Check sheet for the modelled part. Datum: model origin and axes. Units: mm. A direction names the side the tool comes from. Coordinates: 2 decimals unless noted, no trailing zeros. Order: outer loops, then holes, each group sorted by start corner. A loop starts at its lowest first (then second) coordinate and runs counter-clockwise, first axis right, second up.
from build123d import *

# Parameters (mm, degrees)
SKETCH5_W           = 107.15
SKETCH5_H           = 18.5
BOSS_EXTRUDE1_DEPTH = 107.94999
SKETCH4_W           = 77.94999
SKETCH4_H           = 77.15084
CUT_EXTRUDE1_DEPTH  = 7.5
FILLET1_R           = 5
FILLET3_R           = 20
CHAMFER1_SIZE       = 10
CHAMFER1_SIZE2      = 5
CUT_EXTRUDE2_DEPTH  = 2
FILLET4_R           = 20
FILLET5_R           = 2
CUT_EXTRUDE3_START  = -7.5
CUT_EXTRUDE3_DEPTH  = 7.5


with BuildPart() as part:
    # Sketch5 → Boss-Extrude1 (new body)
    with BuildSketch(Plane.ZY.offset(-91.769)):
        with Locations((-38.2134, -9.25)):
            Rectangle(SKETCH5_W, SKETCH5_H)
    extrude(amount=BOSS_EXTRUDE1_DEPTH)

    # Sketch4 → Cut-Extrude1 (cut)
    with BuildSketch(Plane(origin=(0, 0, 0), x_dir=(1, 0, 0), z_dir=(0, 1, 0))):
        with Locations((37.794005, 38.21298)):
            Rectangle(SKETCH4_W, SKETCH4_H)
    extrude(amount=-CUT_EXTRUDE1_DEPTH, mode=Mode.SUBTRACT)

    # Fillet1
    fillet1_edges = [part.edges().sort_by_distance(p)[0] for p in [
        (76.769, -3.75, -76.7884),
        (76.769, -3.75, 0.36244),
        (-1.18099, -3.75, 0.36244),
        (-1.18099, -3.75, -76.7884),
    ]]
    fillet(fillet1_edges, radius=FILLET1_R)

    # Fillet3
    fillet3_edges = [part.edges().sort_by_distance(p)[0] for p in [
        (-16.18099, -9.25, -91.7884),
        (-16.18099, -9.25, 15.3616),
        (91.769, -9.25, -91.7884),
        (91.769, -9.25, 15.3616),
    ]]
    fillet(fillet3_edges, radius=FILLET3_R)

    # Chamfer1
    chamfer1_edges = [part.edges().sort_by_distance(p)[0] for p in [
        (37.794005, 0, -91.7884),
        (91.769, 0, -38.2134),
        (-16.18099, 0, -38.2134),
        (37.794005, 0, 15.3616),
        (-10.323125624, 0, -85.930535624),
        (-10.323125624, 0, 9.503735624),
        (85.911135624, 0, 9.503735624),
        (85.911135624, 0, -85.930535624),
    ]]
    chamfer1_side = [part.faces().sort_by_distance(p)[0] for p in [
        (37.794005, 0, 13.840602865),
    ]]
    chamfer(chamfer1_edges, length=CHAMFER1_SIZE, length2=CHAMFER1_SIZE2, reference=chamfer1_side[0])

    # Sketch6 → Cut-Extrude2 (cut)
    with BuildSketch(Plane.XZ.offset(18.5)):
        with BuildLine():
            Line((3.81901, -91.7884), (71.769, -91.7884))
            ThreePointArc((71.769, -91.7884), (85.911135624, -85.930535624), (91.769, -71.7884))
            Line((91.769, -71.7884), (91.769, -4.6384))
            ThreePointArc((91.769, -4.6384), (85.911135624, 9.503735624), (71.769, 15.3616))
            Line((71.769, 15.3616), (3.81901, 15.3616))
            ThreePointArc((3.81901, 15.3616), (-10.323125624, 9.503735624), (-16.18099, -4.6384))
            Line((-16.18099, -4.6384), (-16.18099, -71.7884))
            ThreePointArc((-16.18099, -71.7884), (-10.323125624, -85.930535624), (3.81901, -91.7884))
        make_face()
        with BuildLine():
            Line((3.81901, -79.7884), (71.769, -79.7884))
            ThreePointArc((71.769, -79.7884), (77.425854249, -77.445254249), (79.769, -71.7884))
            Line((79.769, -71.7884), (79.769, -4.6384))
            ThreePointArc((79.769, -4.6384), (77.425854249, 1.018454249), (71.769, 3.3616))
            Line((71.769, 3.3616), (3.81901, 3.3616))
            ThreePointArc((3.81901, 3.3616), (-1.837844249, 1.018454249), (-4.18099, -4.6384))
            Line((-4.18099, -4.6384), (-4.18099, -71.7884))
            ThreePointArc((-4.18099, -71.7884), (-1.837844249, -77.445254249), (3.81901, -79.7884))
        make_face(mode=Mode.SUBTRACT)
    extrude(amount=-CUT_EXTRUDE2_DEPTH, mode=Mode.SUBTRACT)

    # Fillet4
    # the kernel refuses this fillet: 20 mm, written as the material it adds along each edge
    with BuildSketch(Plane(origin=(71.769, -16.5, -4.6384), x_dir=(1, 0, 0), z_dir=(0, 0, -1))) as fillet4_piece_1:
        with BuildLine():
            CenterArc((16.717797887, 20), FILLET4_R, 244.158067237, 25.841932763)
            Line((8, 2), (8, 0))
            Line((8, 0), (16.717797887, 0))
        make_face()
    revolve(axis=Axis((71.769, -16.5, -4.6384), (0, -1, 0)), revolution_arc=90)
    with BuildSketch(Plane(origin=(79.769, -16.5, -71.7884), x_dir=(1, 0, 0), z_dir=(0, 0, 1)), Plane(origin=(-4.18099, -16.5, -4.6384), x_dir=(-1, 0, 0), z_dir=(0, 0, -1))) as fillet4_piece_2:
        with BuildLine():
            CenterArc((8.717797887, -20), FILLET4_R, 90, 25.841932763)
            Line((0, -2), (0, 0))
            Line((0, 0), (8.717797887, 0))
        make_face()
    extrude(amount=67.15)
    with BuildSketch(Plane(origin=(71.769, -16.5, -71.7884), x_dir=(0, 0, -1), z_dir=(-1, 0, 0))) as fillet4_piece_3:
        with BuildLine():
            CenterArc((16.717797887, 20), FILLET4_R, 244.158067237, 25.841932763)
            Line((8, 2), (8, 0))
            Line((8, 0), (16.717797887, 0))
        make_face()
    revolve(axis=Axis((71.769, -16.5, -71.7884), (0, -1, 0)), revolution_arc=90)
    with BuildSketch(Plane(origin=(3.81901, -16.5, -79.7884), x_dir=(0, 0, -1), z_dir=(1, 0, 0)), Plane(origin=(71.769, -16.5, 3.3616), x_dir=(0, 0, 1), z_dir=(-1, 0, 0))) as fillet4_piece_4:
        with BuildLine():
            CenterArc((8.717797887, -20), FILLET4_R, 90, 25.841932763)
            Line((0, -2), (0, 0))
            Line((0, 0), (8.717797887, 0))
        make_face()
    extrude(amount=67.94999)
    with BuildSketch(Plane(origin=(3.81901, -16.5, -71.7884), x_dir=(-1, 0, 0), z_dir=(0, 0, 1))) as fillet4_piece_5:
        with BuildLine():
            CenterArc((16.717797887, 20), FILLET4_R, 244.158067237, 25.841932763)
            Line((8, 2), (8, 0))
            Line((8, 0), (16.717797887, 0))
        make_face()
    revolve(axis=Axis((3.81901, -16.5, -71.7884), (0, -1, 0)), revolution_arc=90)
    with BuildSketch(Plane(origin=(3.81901, -16.5, -4.6384), x_dir=(0, 0, 1), z_dir=(1, 0, 0))) as fillet4_piece_6:
        with BuildLine():
            CenterArc((16.717797887, 20), FILLET4_R, 244.158067237, 25.841932763)
            Line((8, 2), (8, 0))
            Line((8, 0), (16.717797887, 0))
        make_face()
    revolve(axis=Axis((3.81901, -16.5, -4.6384), (0, -1, 0)), revolution_arc=90)

    # Fillet5
    fillet5_edges = [part.edges().sort_by_distance(p)[0] for p in [
        (-10.323125624, -16.5, -85.930535624),
        (-16.18099, -16.5, -38.2134),
        (-10.323125624, -16.5, 9.503735624),
        (37.794005, -16.5, 15.3616),
        (85.911135624, -16.5, 9.503735624),
        (91.769, -16.5, -38.2134),
        (85.911135624, -16.5, -85.930535624),
        (37.794005, -16.5, -91.7884),
        (-6.18099, 0, -38.2134),
        (-3.252057812, 0, -78.859467812),
        (-3.252057812, 0, 2.432667812),
        (37.794005, 0, -81.7884),
        (37.794005, 0, 5.3616),
        (78.840067812, 0, -78.859467812),
        (78.840067812, 0, 2.432667812),
        (81.769, 0, -38.2134),
        (91.769, -5, -38.2134),
        (85.911135624, -5, 9.503735624),
        (85.911135624, -5, -85.930535624),
        (37.794005, -5, 15.3616),
        (37.794005, -5, -91.7884),
        (-10.323125624, -5, 9.503735624),
        (-10.323125624, -5, -85.930535624),
        (-16.18099, -5, -38.2134),
    ]]
    fillet(fillet5_edges, radius=FILLET5_R)

    # Sketch8 → Cut-Extrude3 (cut)
    with BuildSketch(Plane(origin=(0, -7.5, 0), x_dir=(1, 0, 0), z_dir=(0, 1, 0)).offset(CUT_EXTRUDE3_START)):
        with BuildLine():
            Line((-1.18099, 71.7884), (-1.18099, 4.63756))
            ThreePointArc((-1.18099, 4.63756), (0.283476094, 1.102026094), (3.81901, -0.36244))
            Line((3.81901, -0.36244), (71.769, -0.36244))
            ThreePointArc((71.769, -0.36244), (75.304533906, 1.102026094), (76.769, 4.63756))
            Line((76.769, 4.63756), (76.769, 71.7884))
            ThreePointArc((76.769, 71.7884), (75.304533906, 75.323933906), (71.769, 76.7884))
            Line((71.769, 76.7884), (3.81901, 76.7884))
            ThreePointArc((3.81901, 76.7884), (0.283476094, 75.323933906), (-1.18099, 71.7884))
        make_face()
    extrude(amount=CUT_EXTRUDE3_DEPTH, mode=Mode.SUBTRACT)


solid = part.part
(1) Cross-section at A-A (y = -12). Enter the section's corners in (x, z).
Filled in:
outline: (-16.18, -71.79) arc R20 ccw to (3.82, -91.79) - (71.77, -91.79) arc R20 ccw to (91.77, -71.79) - (91.77, -4.64) arc R20 ccw to (71.77, 15.36) - (3.82, 15.36) arc R20 ccw to (-16.18, -4.64) - close; hole (-1.18, -71.79) arc R5 ccw to (3.82, -76.79) - (71.77, -76.79) arc R5 ccw to (76.77, -71.79) - (76.77, -4.64) arc R5 ccw to (71.77, 0.36) - (3.82, 0.36) arc R5 ccw to (-1.18, -4.64) - close
(2) Cross-section at B-B (z = -48.5). Enter the section's corners in (x, y).
Filled in:
outline: (-16.18, -14.5) arc R2 ccw to (-14.18, -16.5) - (-12.9, -16.5) arc R20 cw to (-4.18, -18.5) - (79.77, -18.5) arc R20 cw to (88.49, -16.5) - (89.77, -16.5) arc R2 ccw to (91.77, -14.5) - (91.77, -6.24) arc R2 ccw to (90.66, -4.45) - (82.19, -0.21) arc R2 ccw to (81.3, 0) - (76.77, 0) - (76.77, -15) - (-1.18, -15) - (-1.18, 0) - (-5.71, 0) arc R2 ccw to (-6.6, -0.21) - (-15.08, -4.45) arc R2 ccw to (-16.18, -6.24) - close
(3) Go/stop test with a flat-tipped pin: P1, Ø6, axis at x = 22, z = -3, coming from the +Y side. Record where the tip stops, or that it passes through.
Filled in:
P1: stops at y = -15
(4) Cross-section at C-C (x = 67.5). Enter the section's corners in (y, z).
Filled in:
outline: (-18.5, -79.79) arc R20 cw to (-16.5, -88.51) - (-16.5, -89.79) arc R2 ccw to (-14.5, -91.79) - (-6.24, -91.79) arc R2 ccw to (-4.45, -90.68) - (-0.21, -82.21) arc R2 ccw to (0, -81.32) - (0, -76.79) - (-15, -76.79) - (-15, 0.36) - (0, 0.36) - (0, 4.89) arc R2 ccw to (-0.21, 5.78) - (-4.45, 14.26) arc R2 ccw to (-6.24, 15.36) - (-14.5, 15.36) arc R2 ccw to (-16.5, 13.36) - (-16.5, 12.08) arc R20 cw to (-18.5, 3.36) - close
(5) Thickness scan on probe 1 along Z at (x, y) = (40.5, -6.25); probe 2 along X at (y, z) = (-14.75, -18); probe 3 along Y at (x, z) = (14, -2). Record the ranges inside material, lowest first.
Filled in:
probe 1: z = -91.79 to -76.79, 0.36 to 15.36
probe 2: x = -16.17 to -1.18, 76.77 to 91.75
probe 3: y = -18.5 to -15
(6) Tool access check on faces 1 (the cylindrical face through (84.08, -16.99, -38.68)), 2 (the flat face through (37, -15, -39)). Record the directions out of +Z, -Z, +X, -X, +Y, -Y that give a thin tool (end or side, any length) a straight path to the whole face; none if there is none.
Filled in:
face 1: +Z, -Z, +X, -Y
face 2: +Y
(7) Release check for a two-part mould opening along Z. For faces 3 (the flat face through (38.27, -2.36, -86.51)), 4 (the flat face through (-10.9, -2.36, -38.68)), 5 (the flat face through (-1.181, -7, -38)) record: +Z half, -Z half, draft (parallel to the pull), parting line (faces both ways), or undercut.
Filled in:
face 3: -Z half
face 4: draft
face 5: undercut
